The listing builds one solid part. Answer for the finished solid, in the listing's coordinates (mm). A direction names the side the tool comes from. Coordinates: 2 decimals unless noted, no trailing zeros. Order: outer loops, then holes, each group sorted by start corner. A loop starts at its lowest first (then second) coordinate and runs counter-clockwise, first axis right, second up. Notation, with made-up numbers: (51, -6) -> (62, -6) arc R25 ccw to (62, 15) -> close; hole circle Ø5 at (35, 17). An arc over 180 degrees is marked (long way). Answer in a Markdown table with one row per item.
```python
from build123d import *

# Parameters (mm, degrees)
SKETCH1_W           = 600
SKETCH1_H           = 300
BOSS_EXTRUDE1_DEPTH = 120
SKETCH3_R           = 10
BOSS_EXTRUDE3_DEPTH = 75
BOSS_EXTRUDE4_START = 75
SKETCH2_R           = 10
BOSS_EXTRUDE4_DEPTH = 75


with BuildPart() as part:
    # Sketch1 → Boss-Extrude1 (new body)
    with BuildSketch(Plane(origin=(0, 0, 0), x_dir=(1, 0, 0), z_dir=(0, 1, 0))):
        Rectangle(SKETCH1_W, SKETCH1_H)
    extrude(amount=BOSS_EXTRUDE1_DEPTH)

    # Sketch3 → Boss-Extrude3 (add)
    with BuildSketch(Plane.XY.offset(150)):
        with Locations(Location((-200, 60, 0), (0, 0, 180))):
            Circle(SKETCH3_R)
        with Locations(Location((200, 60, 0), (0, 0, 180))):
            Circle(SKETCH3_R)
    extrude(amount=BOSS_EXTRUDE3_DEPTH)

    # Sketch2 → Boss-Extrude4 (add)
    with BuildSketch(Plane(origin=(0, 0, -150), x_dir=(-1, 0, 0), z_dir=(0, 0, -1)).offset(BOSS_EXTRUDE4_START)):
        with Locations((-200, 60)):
            Circle(SKETCH2_R)
        with Locations((200, 60)):
            Circle(SKETCH2_R)
    extrude(amount=-BOSS_EXTRUDE4_DEPTH)


solid = part.part
```
(1) For a pull along X with two mould halves and no side action, classify faces 1 (the flat face through (-200, 60, -225)), 2 (the cylindrical face through (190.763, 63.83, 186.975)), 3 (the flat face through (300, 59, 2)) as released by +X, released by -X, zero draft, split by the parting line, or undercut.
Check values:
| item | result |
|---|---|
| face 1 | zero draft |
| face 2 | undercut |
| face 3 | released by +X |
(2) A cutting plane is placed at A-A, the plane y = 60. Determine the outline of the cut face in (x, z), then the cut area to 3 significant figures.
Check values:
| item | result |
|---|---|
| outline | (-300, -150) -> (-210, -150) -> (-210, -225) -> (-190, -225) -> (-190, -150) -> (190, -150) -> (190, -225) -> (210, -225) -> (210, -150) -> (300, -150) -> (300, 150) -> (210, 150) -> (210, 225) -> (190, 225) -> (190, 150) -> (-190, 150) -> (-190, 225) -> (-210, 225) -> (-210, 150) -> (-300, 150) -> close |
| area | 186,000 mm² |
(3) Find the intervals of material crossed by line 1 along Z through (x, y) = (-225.5, 65); line 2 along X through (y, z) = (51, 186), in increasing order. Write a range as from..to.
Check values:
| item | result |
|---|---|
| line 1 | -150..150 |
| line 2 | -204.36..-195.64, 195.64..204.36 |
(4) A cutting plane is placed at B-B, the plane x = 200. Determine the outline of the cut face in (y, z).
Check values:
| item | result |
|---|---|
| outline | (0, -150) -> (50, -150) -> (50, -225) -> (70, -225) -> (70, -150) -> (120, -150) -> (120, 150) -> (70, 150) -> (70, 225) -> (50, 225) -> (50, 150) -> (0, 150) -> close |
(5) Flat-ended cylindrical pins translate along their axes: pin 1 (2 mm diameter, centred on x = 84, y = 22.5, fed in from +Z); pin 2 (6 mm diameter, centred on x = -25, y = 78.5, fed in from -Z); pin 3 (2 mm diameter, centred on x = 193, z = -166.5, fed in from -Y). Find the tip coordinate at first contact, or state that the pin passes through.
Check values:
| item | result |
|---|---|
| pin 1 | z = 150 |
| pin 2 | z = -150 |
| pin 3 | y = 52 |
(6) A cutting plane is placed at C-C, the plane x = 83. Determine the outline of the cut face in (y, z).
Check values:
| item | result |
|---|---|
| outline | (0, -150) -> (120, -150) -> (120, 150) -> (0, 150) -> close |
(7) Which of the six approach directions +Z, -Z, +X, -X, +Y, -Y give full straight-line access (tool end or side, diameter ignored) to faces 4 (the cylindrical face through (-209.237, 63.83, 186.975)), 5 (the flat face through (-300, 59, 2)), 6 (the cylindrical face through (-209.237, 56.17, -188.025))?
Check values:
| item | result |
|---|---|
| face 4 | +Z |
| face 5 | +Z, -Z, -X, +Y, -Y |
| face 6 | -Z |
